Input: dimensioned drawing with shaded views. Units: mm. Origin: part minimum x, y, z. Coordinates: 2 decimals unless noted, no trailing zeros. Write each loop counter-clockwise with the first axis right and the second up, starting at its lowest first coordinate (ties: lowest second). Pieces come first, ordered by that corner, then holes. Notation, with made-up numbers: (26, 18) -> (44, 18) arc R18 ccw to (44, 40) -> close; hole circle Ø9 at (30.5, -7.5). An arc over 180 degrees is marked (long way). One line per item, written item: value. Start each with the question number.
1. Section query D-D, the plane x = 82.55. Output: boundary loops of the cut face in (y, z), and give its area (3 significant figures).
2. Line query: line 1 (X direction, y = 31.5, z = 29) (1 decimal); line 2 (X direction, y = 47, z = 18) (1 decimal); line 3 (Z direction, x = 82.55, y = 37.5). Output: solid intervals per line, ascending.
3. First-contact query: P1, Ø1.7, axis at x = 46, y = 15, coming from the +Z side; P2, Ø3, axis at x = 44.5, y = 32.5, coming from the -Z side; P3, Ø1.5, axis at y = 39, z = 15.5, coming from the +X side (1 decimal); P4, Ø1.5, axis at x = 16.5, z = 30.5, coming from the +Y side. Flat tips, straight axial feed; report the tip coordinate or a pass-through.
4. Mould query, pull axis X, two halves, no side actions, for the marked faces 1, 2, 3 and 4. Classes: released by +X, released by -X, zero draft, split by the parting line, or undercut.
5. Section query B-B, the plane x = 35. Output: boundary loops of the cut face in (y, z), and give its area (4 significant figures).
6. Section query C-C, the plane z = 38. State how many separate pieces and enclosed holes the cut face has, and give its area (3 significant figures).
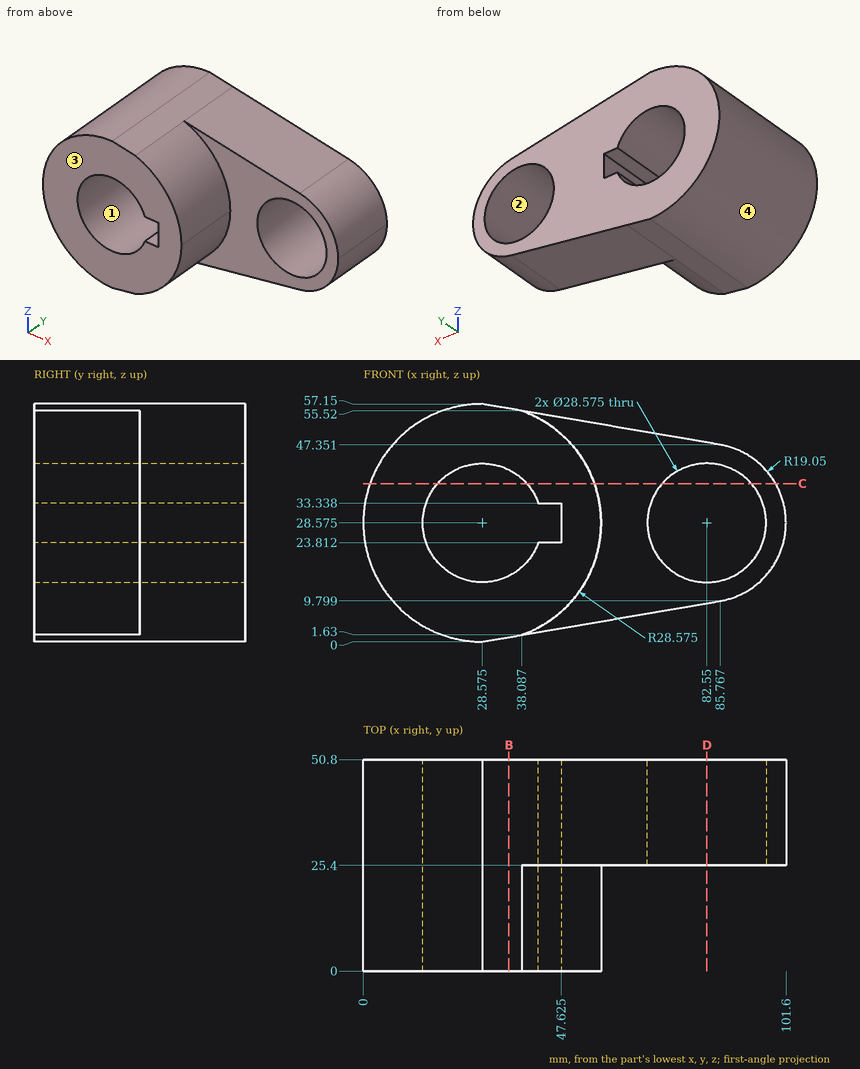
Computed values:
1. outline: (25.4, 9.25) -> (50.8, 9.25) -> (50.8, 14.29) -> (25.4, 14.29) -> close; (25.4, 42.86) -> (50.8, 42.86) -> (50.8, 47.9) -> (25.4, 47.9) -> close
1. area: 256 mm²
2. line 1: x = 0 to 14.3, 47.6 to 68.3, 96.8 to 101.6
2. line 2: x = 2 to 19, 38.2 to 72.9, 92.2 to 98.4
2. line 3: z = 9.25 to 14.29, 42.86 to 47.9
3. P1: stops at z = 51.85
3. P2: stops at z = 2.47
3. P3: stops at x = 97.1
3. P4: passes through
4. face 1: undercut
4. face 2: undercut
4. face 3: zero draft
4. face 4: released by -X
5. outline: (0, 1.1) -> (50.8, 1.1) -> (50.8, 15.81) -> (0, 15.81) -> close; (0, 41.34) -> (50.8, 41.34) -> (50.8, 56.05) -> (0, 56.05) -> close
5. area: 1,495 mm²
6. separate pieces: 3
6. enclosed holes: 0
6. area: 2,210 mm²
